```python
from build123d import *


with BuildPart() as part:
    # Sketch1 → Revolve1 (revolve)
    with BuildSketch(Plane(origin=(0, 0, 0), x_dir=(0, 0, -1), z_dir=(1, 0, 0)), mode=Mode.PRIVATE) as revolve1_sk:
        with BuildLine():
            Line((-9, 52.4), (-8.1, 52.4))
            Line((-8.1, 52.4), (-5.961624878, 46.638267033))
            ThreePointArc((-5.961624878, 46.638267033), (-4.902735476, 45.99360404), (-4.030378188, 46.87441611))
            Line((-4.030378188, 46.87441611), (-3.6, 50.7))
            Line((-3.6, 50.7), (0, 50.7))
            Line((0, 50.7), (0, 45))
            Line((0, 45), (-6.8, 45))
            Line((-6.8, 45), (-9, 52.4))
        make_face()
    revolve(revolve1_sk.sketch.rotate(Axis((0, 0, 0), (0, 0, -1)), 90), axis=Axis((0, 0, 0), (0, 0, -1)))


solid = part.part
```
The model under review builds one solid part; all positions refer to its coordinate system, in mm. A direction names the side the tool comes from. Round coordinates to 2 decimals unless told otherwise and drop trailing zeros. Loops run counter-clockwise (first coordinate to the right, second up) from the corner with the lowest first, then second, coordinate; pieces in that order, holes last. Notation, with made-up numbers: (-31.75, 22) - (17.25, 22) arc R31 ccw to (17.25, 60) - close; hole circle Ø10 at (63.5, 77.25). An arc over 180 degrees is marked (long way). Use a Markdown table: item, result. Add a question column.
Q1. For probe 1 along Y at (x, z) = (0, 3.25); probe 2 along Z at (x, y) = (41, 23.5); probe 3 along X at (y, z) = (8.5, 0.5), list the stretches that pass through material, from the lowest coordinate up.
Q2. Machinability: for faces 4 (the face through (-37.233, 28.549, 6.065)), 5 (the face through (48.36, -15.23, 1.77)), 6 (the face through (-38.621, -35.414, 8.544)), which of the approach directions +Z, -Z, +X, -X, +Y, -Y give a long, thin tool a straight path to every point of the face, cutting with its end or side? Answer none if there is none.
Q3. Add section A-A (y = 0). State the section outline as (x, z) points.
Q4. Add section B-B (z = 1.5). State the section outline as (x, y) points.
Q5. Insertion check: pin 1 Ø5 at (y, z) = (7.5, 3) entering from -X; pin 2 Ø1.5 at (y, z) = (-13.5, 4) entering from -X; pin 3 Ø3 at (y, z) = (10, 2) entering from -X. Each pin has a flat end and moves straight along its axis. Give the tip position at first contact, or say it passes through.
Q6. The part is to be moulded in two halves that separate along Y. For faces 1 (the face through (-19, 41, 0)), 2 (the face through (20.765, 39.923, 3.448)), 3 (the face through (-10.213, 45.993, 4.003)), say which applies: pulls with the +Y half, pulls with the -Y half, needs draft (parallel to the pull), parting line crosses it, or undercut.
Worked answers:
| question | item | result |
|---|---|---|
| 1 | probe 1 | -50.7 to -45, 45 to 50.7 |
| 1 | probe 2 | 0 to 3.99, 6.19 to 7.47 |
| 1 | probe 3 | -49.98 to -44.19, 44.19 to 49.98 |
| 2 | face 4 | none |
| 2 | face 5 | -Z |
| 2 | face 6 | +Z, -Z |
| 3 | outline | (-52.4, 8.1) - (-46.64, 5.96) arc R1 cw to (-46.87, 4.03) - (-50.7, 3.6) - (-50.7, 0) - (-45, 0) - (-45, 6.8) - (-52.4, 9) - close; (45, 0) - (50.7, 0) - (50.7, 3.6) - (46.87, 4.03) arc R1 cw to (46.64, 5.96) - (52.4, 8.1) - (52.4, 9) - (45, 6.8) - close |
| 4 | outline | circle Ø101.4 at (0, 0); hole circle Ø90 at (0, 0) |
| 5 | pin 1 | x = -50.45 |
| 5 | pin 2 | x = -49.04 |
| 5 | pin 3 | x = -49.98 |
| 6 | face 1 | needs draft |
| 6 | face 2 | undercut |
| 6 | face 3 | parting line crosses it |
